Can you work these out from the drawing? Everything is in mm from the part's minimum corner. A direction names the side the tool comes from. Give positions to 0.01 mm unless a question says otherwise; leave off trailing zeros. Write each loop counter-clockwise with the first axis right and the second up, starting at its lowest first coordinate (ties: lowest second). Pieces come first, ordered by that corner, then holes. Notation, with made-up numbers: (73.5, -29.5) -> (77.5, -29.5) arc R23 cw to (77.5, 8.5) -> close; hole circle Ø3 at (-35.5, -3.5). An arc over 180 degrees is marked (long way). Write item = value, one per line. Start each with the question number.
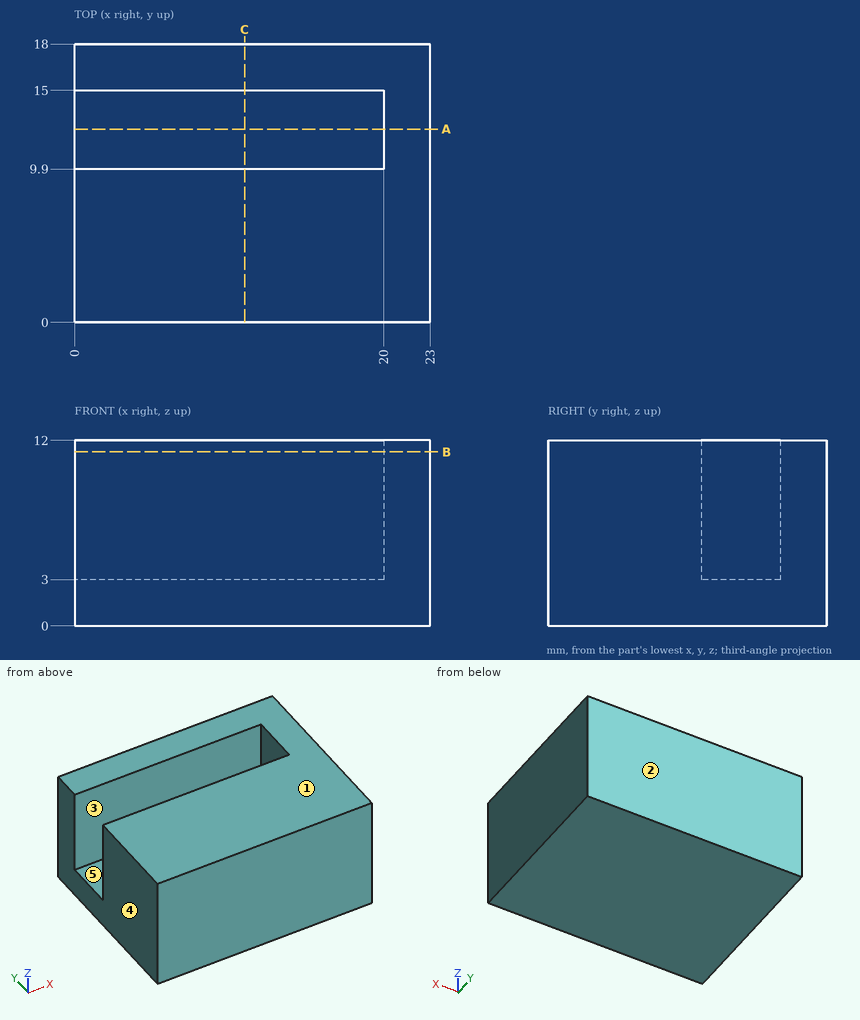
(1) I'm going to push flat-ended pins straight in: pin 1 (5 mm diameter, centred on y = 8, z = 9.5, fed in from -X); pin 2 (2.5 mm diameter, centred on y = 13, z = 8, fed in from -X). Where does each tip first touch, or does it pass through?
(2) If I drill on line 1 along Y through (x, z) = (4, 8.5); line 2 along Z through (x, y) = (13.25, 13); line 3 along X through (y, z) = (13.75, 7.5), over which ranges is the centre line in solid material (lowest first)? Write a range as from..to.
(3) Imagine slicing it at A-A (y = 12.5). Please give me the cut outline in (x, z), then the cut area to 3 significant figures.
(4) Imagine slicing it at B-B (z = 11.25). Please give me the cut outline in (x, y), then the cut area to 3 significant figures.
(5) Imagine slicing it at C-C (x = 11). Please give me the cut outline in (y, z).
(6) On a 3-axis mill with a long thin cutter (end or side, diameter ignored), from which of +Z, -Z, +X, -X, +Y, -Y can I reach the whole of each face in a straight line? I mean the marked faces 4 and 5. Say none if no direction works.
(7) We'd pull the mould along Y, two halves only. Please class the marked faces 1, 2 and 3: released by +Y, released by -Y, zero draft, split by the parting line, or undercut.
Answers below:
q1.pin_1 = 0
q1.pin_2 = 20
q2.line_1 = 0..9.9, 15..18
q2.line_2 = 0..3
q2.line_3 = 20..23
q3.outline = (0, 0) -> (23, 0) -> (23, 12) -> (20, 12) -> (20, 3) -> (0, 3) -> close
q3.area = 96.0 mm^2
q4.outline = (0, 0) -> (23, 0) -> (23, 18) -> (0, 18) -> (0, 15) -> (20, 15) -> (20, 9.9) -> (0, 9.9) -> close
q4.area = 312 mm^2
q5.outline = (0, 0) -> (18, 0) -> (18, 12) -> (15, 12) -> (15, 3) -> (9.9, 3) -> (9.9, 12) -> (0, 12) -> close
q6.face_4 = +Z, -Z, -X, +Y, -Y
q6.face_5 = +Z, -X
q7.face_1 = zero draft
q7.face_2 = released by +Y
q7.face_3 = undercut
